Design review of the part built by this model. Coordinates are the model's own, in mm. A direction names the side the tool comes from. Coordinates: 2 decimals unless noted, no trailing zeros. Loops run counter-clockwise (first coordinate to the right, second up) from the corner with the lowest first, then second, coordinate; pieces in that order, holes last.
Autodesk Inventor part; units mm, degrees
ref_plane "YZ Plane" through (0, 0, 0) normal (1, 0, 0) x (0, 1, 0)
ref_plane "XZ Plane" through (0, 0, 0) normal (0, 1, 0) x (-1, 0, 0)
ref_plane "XY Plane" through (0, 0, 0) normal (0, 0, 1) x (1, 0, 0)
sketch "Sketch1" plane through (0, 0, 0) normal (1, 0, 0) x (0, 1, 0)
  line L0 (0, 0) -> (0, -7.42)
  line L1 (0, -7.42) -> (1.0563, -7.42)
  line L2 (1.0563, -7.42) -> (2.51, -2.84)
  line L3 (2.51, -2.84) -> (6.31, -2.84)
  line L4 (6.31, -2.84) -> (6.31, -8.45)
  line L5 (6.31, -8.45) -> (10.81, -8.45)
  line L6 (10.81, -8.45) -> (10.81, -3.65)
  line L7 (10.81, -3.65) -> (10.17, -3.65)
  line L8 (10.17, -3.65) -> (10.17, 0)
  line L9 (0, 0) -> (9.5063, 0) construction
  line L10 (0, 0) -> (0, 7.42)
  line L11 (0, 7.42) -> (1.0563, 7.42)
  line L12 (1.0563, 7.42) -> (2.51, 2.84)
  line L13 (2.51, 2.84) -> (6.31, 2.84)
  line L14 (6.31, 2.84) -> (6.31, 8.45)
  line L15 (6.31, 8.45) -> (10.81, 8.45)
  line L16 (10.81, 8.45) -> (10.81, 3.65)
  line L17 (10.81, 3.65) -> (10.17, 3.65)
  line L18 (10.17, 3.65) -> (10.17, 0)
  dimension "d0" = 8.45
  dimension "d1" = 4.5
  dimension "d2" = 0.64
  dimension "d3" = 3.8
  dimension "d4" = 7.42
  dimension "d5" = 3.65
  dimension "d6" = 10.81
  dimension "d7" = 2.84
extrude "Extrusion1" add sketch "Sketch1" against normal blind 135
sketch "Sketch2" plane through (0, 10.17, 3.65) normal (0, 1, 0) x (1, 0, 0)
  line L0 (0, 3.65) -> (-10, 3.65) construction
  circle A0 centre (-10, 3.65) radius 1.615
  dimension "d10" = 3.23
  dimension "d11" = 10
extrude "Extrusion2" cut sketch "Sketch2" against normal blind 30
sketch "Sketch3" plane through (0, 10.17, 3.65) normal (0, 1, 0) x (1, 0, 0)
  circle A0 centre (-10, 3.65) radius 1.615
  circle A1 centre (-10, 3.65) radius 2.9
  point P0 (0, 3.65)
  dimension "d14" = 5.8
extrude "Extrusion3" cut sketch "Sketch3" against normal blind 3.5
pattern_linear "Rectangular Pattern1" count 8 spacing 40 along (-1, 0, 0) of "Extrusion3", "Extrusion2"
properties part number "Rail"
Q1. Take a section at D-D, the plane x = -69. Write out the cut boundary in (y, z).
Q2. Take a section at A-A, the plane y = 8. Write out the cut boundary in (x, z), then the cut area to 3 significant figures.
Q3. Machinability: for faces 5 (the cylindrical face through (-132.9, 8.4, -0.1)), 6 (the flat face through (-67, 6.31, 6)), 7 (the flat face through (-67, 10.81, -6)), 8 (the flat face through (-67, 6.31, -6)), 9 (the flat face through (-67, 9, 8.45)), which of the approach directions +Z, -Z, +X, -X, +Y, -Y give a long, thin tool a straight path to every point of the face, cutting with its end or side? Answer none if there is none.
Q4. The part is to be moulded in two halves that separate along Z. For faces 1 (the flat face through (-67, 9, -8.45)), 2 (the cylindrical face through (-91.613, 3.382, -0.071)), 3 (the flat face through (-48.75, 6.67, 1.25)), 4 (the flat face through (-67, 4, 2.84)), say which applies: pulls with the +Z half, pulls with the -Z half, needs draft (parallel to the pull), parting line crosses it, or undercut.
Q5. For line 1 (X direction, y = 7.5, z = 0); line 2 (X direction, y = 3.5, z = 0) (3 decimals); line 3 (Z direction, x = -10, y = 5) (3 decimals), list the stretches that pass through material, from the lowest coordinate up.
Q6. Take a section at B-B, the plane x = -50. Write out the cut boundary in (y, z) (3 decimals).
Q7. Clearance check with flat-ended pins moving along their axes: pin 1 Ø3.5 at (x, z) = (-10, 0) entering from -Y; pin 2 Ø5 at (x, z) = (-130, 0) entering from +Y; pin 3 Ø1.9 at (x, y) = (-53, 3.5) entering from +Z; pin 4 Ø0.8 at (x, y) = (-64, 0.5) entering from +Z. State where each tip first meets the part, or that it passes through.
Q8. Take a section at C-C, the plane z = -6.25. Write out the cut boundary in (x, y), then the cut area to 3 significant figures.
Entries:
1. outline: (0, -7.42) - (1.06, -7.42) - (2.51, -2.84) - (6.31, -2.84) - (6.31, -8.45) - (10.81, -8.45) - (10.81, -3.65) - (10.17, -3.65) - (10.17, 3.65) - (10.81, 3.65) - (10.81, 8.45) - (6.31, 8.45) - (6.31, 2.84) - (2.51, 2.84) - (1.06, 7.42) - (0, 7.42) - close
2. outline: (-135, -8.45) - (0, -8.45) - (0, 8.45) - (-135, 8.45) - close; hole circle Ø5.8 at (-130, 0); hole circle Ø5.8 at (-90, 0); hole circle Ø5.8 at (-50, 0); hole circle Ø5.8 at (-10, 0)
2. area: 2,180 mm2
3. face 5: +Y
3. face 6: +Z, +X, -X
3. face 7: +Z, -Z, +X, -X, +Y
3. face 8: -Z, +X, -X
3. face 9: +Z, +X, -X, +Y, -Y
4. face 1: pulls with the -Z half
4. face 2: undercut
4. face 3: undercut
4. face 4: pulls with the +Z half
5. line 1: x = -135 to -132.9, -127.1 to -92.9, -87.1 to -52.9, -47.1 to -12.9, -7.1 to 0
5. line 2: x = -135 to -131.615, -128.385 to -91.615, -88.385 to -51.615, -48.385 to -11.615, -8.385 to 0
5. line 3: z = -2.84 to -1.615, 1.615 to 2.84
6. outline: (0, -7.42) - (1.056, -7.42) - (2.51, -2.84) - (6.31, -2.84) - (6.31, -8.45) - (10.81, -8.45) - (10.81, -3.65) - (10.17, -3.65) - (10.17, -2.9) - (6.67, -2.9) - (6.67, -1.615) - (0, -1.615) - close; (0, 1.615) - (6.67, 1.615) - (6.67, 2.9) - (10.17, 2.9) - (10.17, 3.65) - (10.81, 3.65) - (10.81, 8.45) - (6.31, 8.45) - (6.31, 2.84) - (2.51, 2.84) - (1.056, 7.42) - (0, 7.42) - close
7. pin 1: stops at y = 0
7. pin 2: stops at y = 6.67
7. pin 3: stops at z = 2.84
7. pin 4: stops at z = 7.42
8. outline: (-135, 0) - (0, 0) - (0, 1.43) - (-135, 1.43) - close; (-135, 6.31) - (0, 6.31) - (0, 10.81) - (-135, 10.81) - close
8. area: 800 mm2
